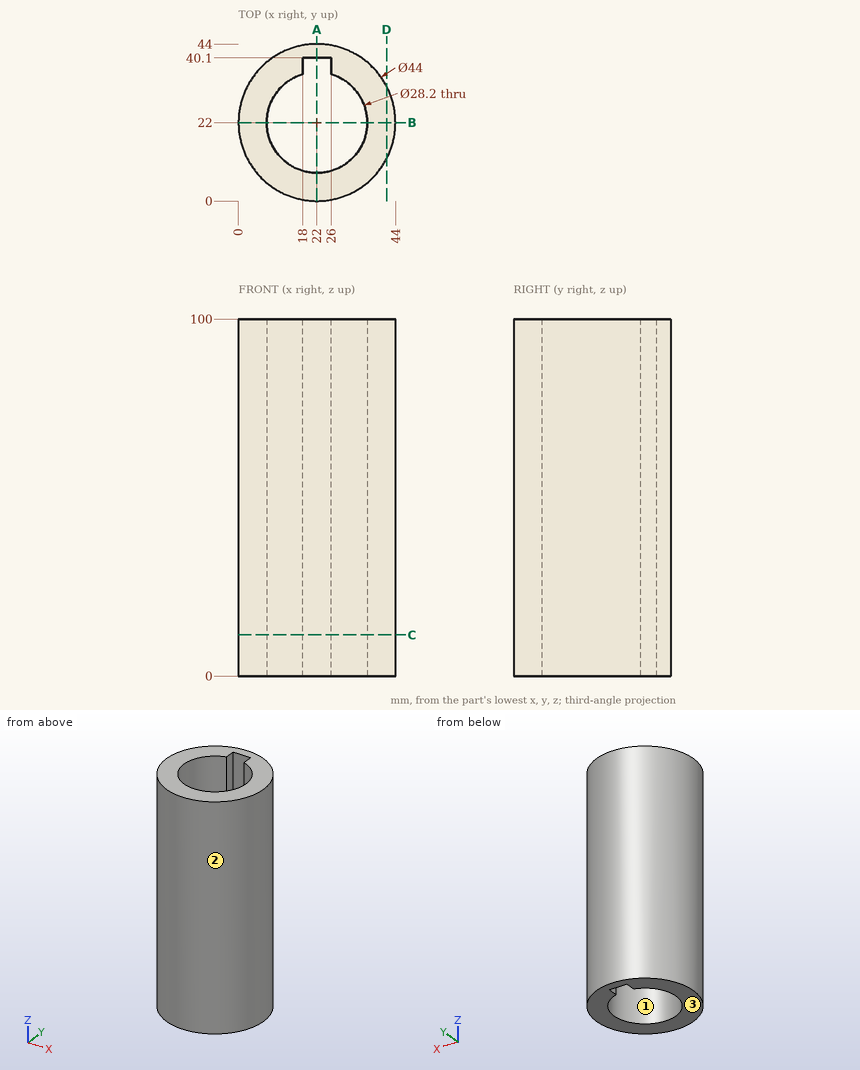
Can you work these out from the drawing? Everything is in mm from the part's minimum corner. Give positions to 0.01 mm unless a question says otherwise; leave off trailing zeros. Loops run counter-clockwise (first coordinate to the right, second up) from the corner with the lowest first, then second, coordinate; pieces in that order, holes last. Notation, with made-up numbers: M -34.75,56.25 L -29.75,56.25 A28 cw -29.75,81.25 Z; hole C 2.25,4 d8. An arc over 180 degrees is marked long. Use CSV: the item, a comma, the result in double quotes. Start each with the question number.
1. Imagine slicing it at B-B, the plane y = 22. Write out the boundary of the cut face in (x, z), plus the area to 3 significant figures.
2. Imagine slicing it at A-A, the plane x = 22. Write out the boundary of the cut face in (y, z), plus the area to 3 significant figures.
3. If I drill on L1, parallel to Y at x = 22, z = 35; L2, parallel to X at y = 9, z = 89; L3, parallel to Y at x = 13.5, z = 5, over which ranges is the centre line in solid material (lowest first)?
4. Imagine slicing it at C-C, the plane z = 11.5. Write out the boundary of the cut face in (x, y).
5. If we mould it in two halves opening along Y, with no side actions, what happens to the marked faces 1, 2 and 3? For each: released by +Y, released by -Y, zero draft, split by the parting line, or undercut.
6. For P1, Ø2.5, axis at y = 38.5, z = 51.5, coming from the +X side; P2, Ø4, axis at x = 22.5, z = 61, coming from the -Y side; P3, Ø2.5, axis at y = 38, z = 31, coming from the -X side; P4, Ø17, axis at x = 22, y = 22, coming from the -Z side, each with a flat end and sliding along its axis, tell me the tip position at first contact or that it passes through.
7. Imagine slicing it at D-D, the plane x = 41.5. Write out the boundary of the cut face in (y, z), plus the area to 3 significant figures.
Response values:
1,outline,"M 0,0 L 7.9,0 L 7.9,100 L 0,100 Z; M 36.1,0 L 44,0 L 44,100 L 36.1,100 Z"
1,area,"1,580 mm^2"
2,outline,"M 0,0 L 7.9,0 L 7.9,100 L 0,100 Z; M 40.1,0 L 44,0 L 44,100 L 40.1,100 Z"
2,area,"1,180 mm^2"
3,L1,"0 to 7.9, 40.1 to 44"
3,L2,"4.25 to 16.54, 27.46 to 39.75"
3,L3,"1.71 to 10.75, 33.25 to 42.29"
4,outline,"C 22,22 d44; hole M 18,35.52 A14.1 ccw long 26,35.52 L 26,40.1 L 18,40.1 Z"
5,face 1,"undercut"
5,face 2,"split by the parting line"
5,face 3,"zero draft"
6,P1,"x = 37.86"
6,P2,"y = 0"
6,P3,"x = 5.68"
6,P4,"through"
7,outline,"M 11.81,0 L 32.19,0 L 32.19,100 L 11.81,100 Z"
7,area,"2,040 mm^2"
